Part model, mm, in its own coordinate system. A direction names the side the tool comes from. Round coordinates to 2 decimals unless told otherwise and drop trailing zeros. Write each loop counter-clockwise with the first axis right and the second up, starting at its lowest first coordinate (ties: lowest second). Pieces come first, ordered by that corner, then holes.
```python
from build123d import *

# Parameters (mm, degrees)
F0_W     = 20
F0_H     = 20
F0_R     = 2.5
F1_DEPTH = 2


with BuildPart() as f1:
    # F0 (on Top) → F1 (new body)
    with BuildSketch(Plane.XY):
        with Locations((10, -10)):
            Rectangle(F0_W, F0_H)
        with Locations((5, -15)):
            Circle(F0_R, mode=Mode.SUBTRACT)
        with Locations((15, -15)):
            Circle(F0_R, mode=Mode.SUBTRACT)
        with Locations((5, -5)):
            Circle(F0_R, mode=Mode.SUBTRACT)
        with Locations((15, -5)):
            Circle(F0_R, mode=Mode.SUBTRACT)
        with Locations((5, -5)):
            Circle(F0_R)
        with Locations((15, -5)):
            Circle(F0_R)
        with Locations((15, -15)):
            Circle(F0_R)
        with Locations((5, -15)):
            Circle(F0_R)
    extrude(amount=-F1_DEPTH)

    # F0 (on Top) → F4 section 0
    with BuildSketch(Plane.XY, mode=Mode.PRIVATE) as f4_s0:
        with Locations((15, -15)):
            Circle(F0_R)
    loft([f4_s0.sketch, Vertex(15, -15, 12)])

    # F0 (on Top) → F5 section 0
    with BuildSketch(Plane.XY, mode=Mode.PRIVATE) as f5_s0:
        with Locations((15, -5)):
            Circle(F0_R)
    loft([Vertex(15, -5, 12), f5_s0.sketch])

    # F0 (on Top) → F6 section 0
    with BuildSketch(Plane.XY, mode=Mode.PRIVATE) as f6_s0:
        with Locations((5, -5)):
            Circle(F0_R)
    loft([f6_s0.sketch, Vertex(5, -5, 12)])

    # F0 (on Top) → F7 section 0
    with BuildSketch(Plane.XY, mode=Mode.PRIVATE) as f7_s0:
        with Locations((5, -15)):
            Circle(F0_R)
    loft([Vertex(5, -15, 12), f7_s0.sketch])


solid = f1.part
```
Q1. Mould opens along Y. For faces 3 (the flat face through (10, 0, -1)), 4 (the flat face through (10, -10, -2)), 5 (the flat face through (10, -20, -1)), 6 (the conical face through (4.1, -14.1, 5.9)) say: +Y half, -Y half, draft (parallel to the pull), parting line (faces both ways), or undercut.
Values follow:
face 3: +Y half
face 4: draft
face 5: -Y half
face 6: undercut
Q2. Which spindle directions (+Z, -Z, +X, -X, +Y, -Y) get a long thin tool onto all of the face, cutting with end or side? Do faces 1 (the flat face through (0, -10, -1)), 2 (the flat face through (10, -10, 0)). Say none if no direction does.
Values follow:
face 1: +Z, -Z, -X, +Y, -Y
face 2: +Z
Q3. Drop flat-ended pins along their axis: pin 1 (5 mm diameter, centred on y = -2.5, z = 9, fed in from -X); pin 2 (2 mm diameter, centred on y = -8, z = 1.5, fed in from +X); pin 3 (4 mm diameter, centred on x = 14.5, z = 0.5, fed in from +Y); pin 4 (5 mm diameter, centred on y = -3, z = 4.5, fed in from +X). Give the stop position or say it passes through.
Values follow:
pin 1: stops at x = 4.18
pin 2: stops at x = 15.94
pin 3: stops at y = 0
pin 4: stops at x = 16.92
Q4. Wall check: L1, parallel to Z at x = 19, y = -8.5; L2, parallel to Y at x = 6.5, z = 3 (3 decimals); L3, parallel to X at y = -4.75, z = 1.5. Give the ranges that are in metal, low to high.
Values follow:
L1: z = -2 to 0
L2: y = -16.125 to -13.875, -6.125 to -3.875
L3: x = 2.83 to 7.17, 12.83 to 17.17
Q5. Cut at C-C on x = 18. Write the cut outline in (y, z).
Values follow:
outline: (-20, -2) - (0, -2) - (0, 0) - (-20, 0) - close
Q6. Cut at B-B on y = -9. Write the cut outline in (x, z), plus the area to 3 significant figures.
Values follow:
outline: (0, -2) - (20, -2) - (20, 0) - (0, 0) - close
area: 40.0 mm2
Q7. Cut at A-A on z = 0.5. Write the cut outline in (x, y), plus the area to 3 significant figures.
Values follow:
outline: circle Ø4.79 at (5, -15); circle Ø4.79 at (5, -5); circle Ø4.79 at (15, -15); circle Ø4.79 at (15, -5)
area: 72.1 mm2
Q8. Cut at D-D on z = 6.5. Write the cut outline in (x, y).
Values follow:
outline: circle Ø2.29 at (5, -15); circle Ø2.29 at (5, -5); circle Ø2.29 at (15, -15); circle Ø2.29 at (15, -5)
